The model under review builds one solid part; all positions refer to its coordinate system, in mm. Round coordinates to 2 decimals unless told otherwise and drop trailing zeros. Write each loop counter-clockwise with the first axis right and the second up, starting at its lowest first coordinate (ties: lowest second). Pieces come first, ordered by that corner, then holes. Notation, with made-up numbers: M 66,65.25 L 104,65.25 A17 cw 104,98.25 Z; hole C 5,56.5 d1. An arc over 180 degrees is marked long. One line per item, written item: value. Start each with the question number.
1) Take a section at C-C, the plane x = 23. Write out the cut boundary in (y, z), and give its area (3 significant figures).
2) Take a section at B-B, the plane y = 30. Write out the cut boundary in (x, z).
3) Mouldability with a two-part tool opening along X and no side actions: class faces 1 (the face through (20.299, -17.634, -1.479)), 2 (the face through (-58.8, -98.2, -1.5)), 3 (the face through (1, -99.344, -1)), 4 (the face through (58.9, -98.1, -1.5)) as +X half, -X half, draft (parallel to the pull), parting line (faces both ways), or undercut.
4) Take a section at A-A, the plane x = 0. Write out the cut boundary in (y, z).
5) Wall thickness on probe 1 along Y at (x, z) = (0, -1.9); probe 2 along X at (y, z) = (-21.5, -0.15); probe 3 along X at (y, z) = (-80, -0.85): over which ranges is each line inside the solid? List them lowest first.
6) For P1, Ø8, axis at x = 0, y = 30, coming from the +Z side; P2, Ø7, axis at x = 0, y = -80, coming from the -Z side, all flat-tipped, find the tip position at first contact; note any pin that passes through.
Autodesk Inventor part; units mm, degrees
ref_plane "YZ Plane" through (0, 0, 0) normal (1, 0, 0) x (0, 1, 0)
ref_plane "XZ Plane" through (0, 0, 0) normal (0, 1, 0) x (-1, 0, 0)
ref_plane "XY Plane" through (0, 0, 0) normal (0, 0, 1) x (1, 0, 0)
sketch "スケッチ1" plane through (0, 0, 0) normal (0, 0, 1) x (1, 0, 0)
  circle A0 centre (0, 0) radius 21.2
  circle A1 centre (0, 0) radius 7.5
  circle A2 centre (0, 0) radius 30
  circle A3 centre (20.819222, -21.6) radius 22.5
  circle A4 centre (20.819222, -21.6) radius 14
  circle A5 centre (20.819222, -21.6) radius 62
  circle A6 centre (0, -80) radius 48
  circle A7 centre (0, -80) radius 50
  circle A8 centre (20.819222, -21.6) radius 4
  circle A9 centre (0, -80) radius 4
  dimension "d2" = 60
  dimension "d4" = 124
  dimension "d0" = 42.4
  dimension "d1" = 15
  dimension "d3" = 28
  dimension "d5" = 100
  dimension "d23" = 8
  dimension "d41" = 8
sketch "スケッチ2" plane through (0, 0, 0) normal (0, 0, 1) x (1, 0, 0)
  line L0 (0, 0) -> (24.501973, 0) construction
  line L1 (0, 0) -> (12.5, 0) construction
  line L2 (0, 0) -> (10.253048, 10.253048)
  line L3 (0, 0) -> (14.5, 0) construction
  line L4 (10.253048, 10.253048) -> (-10.253048, -10.253048)
  circle A0 centre (10.253048, 10.253048) radius 2
  circle A1 centre (-10.253048, -10.253048) radius 2
  circle A2 centre (0, 0) radius 7.5
  line L5 (0, 0) -> (28.190779, 10.260604)
  line L6 (0, 0) -> (30, 0) construction
  line L7 (0, 0) -> (-28.190779, 10.260604)
  line L8 (0, 0) -> (30, 0) construction
  circle A3 centre (-28.190779, 10.260604) radius 2.5
  line L9 (0, 0) -> (0, 30)
  circle A4 centre (0, 30) radius 2.5
  circle A5 centre (28.190779, 10.260604) radius 2.5
  dimension "d9" = 14.5
  dimension "d10" = 45
  dimension "d11" = 29
  dimension "d12" = 4
  dimension "d13" = 4
  dimension "d14" = 15
  dimension "d15" = 30
  dimension "d16" = 20
  dimension "d17" = 30
  dimension "d18" = 160
  dimension "d19" = 5
  dimension "d20" = 30
  dimension "d21" = 5
  dimension "d22" = 5
sketch "スケッチ3" plane through (0, 0, 0) normal (0, 0, 1) x (1, 0, 0)
  line L0 (60, -99.343647) -> (-60, -99.343647)
  line L1 (-60, -99.343647) -> (-60, 99.343647)
  line L2 (-60, 99.343647) -> (60, 99.343647)
  line L3 (60, 99.343647) -> (60, -99.343647)
  line L4 (60, -99.343647) -> (-60, 99.343647) construction
  line L5 (-60, -99.343647) -> (60, 99.343647) construction
  point P0 (0, 0)
  dimension "d25" = 120
extrude "押し出し1" add sketch "スケッチ3" against normal blind 3
sketch "スケッチ4" plane through (0, 0, 0) normal (0, 0, 1) x (1, 0, 0)
  line L0 (0, 45.071117) -> (68.359536, 45.071117)
  line L1 (68.359536, 45.071117) -> (-74.382402, 45.071117)
  line L2 (-74.382402, 45.071117) -> (108.165644, 45.071117)
  line L3 (108.165644, 45.071117) -> (108.165644, 129.415375)
  line L4 (108.165644, 129.415375) -> (-74.382402, 129.415375)
  line L5 (-74.382402, 129.415375) -> (-74.382402, 45.071117)
  point P0 (0, 0)
extrude "押し出し4" cut sketch "スケッチ4" against normal blind 10
fillet "フィレット1" radius 4 4 edges at (-60, 45.0711, -1.5) (60, 45.0711, -1.5) (-60, -99.3436, -1.5) (60, -99.3436, -1.5)
extrude "押し出し7" cut sketch "スケッチ1" against normal blind 10 contours A8 A2 | A2 A8 | A9 A5 | A5 A9
extrude "押し出し8" cut sketch "スケッチ2" against normal blind 10 contours A0 | A1 | A3 | A4 | A5
properties part number "板"
Checked values:
1. outline: M -99.34,-3 L -24.95,-3 L -24.95,0 L -99.34,0 Z; M -18.25,-3 L 45.07,-3 L 45.07,0 L -18.25,0 Z
1. area: 413 mm2
2. outline: M -60,-3 L -2.5,-3 L -2.5,0 L -60,0 Z; M 2.5,-3 L 60,-3 L 60,0 L 2.5,0 Z
3. face 1: undercut
3. face 2: -X half
3. face 3: draft
3. face 4: +X half
4. outline: M -99.34,-3 L -84,-3 L -84,0 L -99.34,0 Z; M -76,-3 L 27.5,-3 L 27.5,0 L -76,0 Z; M 32.5,-3 L 45.07,-3 L 45.07,0 L 32.5,0 Z
5. probe 1: y = -99.34 to -84, -76 to 27.5, 32.5 to 45.07
5. probe 2: x = -60 to 16.82, 24.82 to 60
5. probe 3: x = -60 to -4, 4 to 60
6. P1: stops at z = 0
6. P2: passes through
